The listing builds one solid part. Answer for the finished solid, in the listing's coordinates (mm). Coordinates: 2 decimals unless noted, no trailing zeros. Write each loop counter-clockwise with the first axis right and the second up, starting at its lowest first coordinate (ties: lowest second). Pieces come first, ordered by that corner, then holes. Notation, with made-up numbers: M 8,-17 L 53,-17 A23 ccw 53,-2 Z; hole C 59.25,84 d6. An arc over 180 degrees is marked long. Put each result on its own line as item: value. Start each with the question number.
```python
from build123d import *

# Parameters (mm, degrees)
SKETCH_1_W             = 25
SKETCH_1_H             = 25
SKETCH_1_W_2           = 19
SKETCH_1_H_2           = 19
EXTRUDE_1_DEPTH        = 1285.5
SKETCH_6_R             = 6
CUT_EXTRUDE_1_DEPTH    = 3
PATTERN_LINEAR_1_COUNT = 2
PATTERN_LINEAR_1_PITCH = 1242.5


with BuildPart() as part:
    # 草图1 → 拉伸1 (new body)
    with BuildSketch(Plane.XY):
        with Locations((12.5, -12.5)):
            Rectangle(SKETCH_1_W, SKETCH_1_H)
        with Locations((12.5, -12.5)):
            Rectangle(SKETCH_1_W_2, SKETCH_1_H_2, mode=Mode.SUBTRACT)
    extrude(amount=EXTRUDE_1_DEPTH)

    # 草图4 → Ø6.0 (6) 直径孔1 (revolve, cut)
    with BuildSketch(Plane(origin=(0, -12.5, 1264), x_dir=(0, 0, 1), z_dir=(0, 1, 0))):
        Polygon((0, 0), (0, 31.802581857), (3, 30), (3, 0), align=None)
    hole_wizard_6_0_6_1 = revolve(axis=Axis((-6.35, -12.5, 1264), (1, 0, 0)), mode=Mode.SUBTRACT)

    # 草图6 → 切除-拉伸1 (cut)
    with BuildSketch(Plane.ZY.offset(-25)):
        with Locations(Location((1264, -12.5, 0), (0, 0, 270))):
            Circle(SKETCH_6_R)
    cut_extrude_1 = extrude(amount=CUT_EXTRUDE_1_DEPTH, mode=Mode.SUBTRACT)

    # 阵列(线性)1: Ø6.0 (6) 直径孔1, 切除-拉伸1 ×2
    with Locations(*[(0, 0, -i * PATTERN_LINEAR_1_PITCH) for i in range(1, PATTERN_LINEAR_1_COUNT)]):
        add(hole_wizard_6_0_6_1, mode=Mode.SUBTRACT)
        add(cut_extrude_1, mode=Mode.SUBTRACT)


solid = part.part
```
1) A cutting plane is placed at B-B on z = 116. Write down the section's boundary in (x, y), then the cut area to 3 significant figures.
2) A cutting plane is placed at A-A on x = 15.5. Write down the section's boundary in (y, z).
3) Straight lines are drawn through the part: probe 1 along X at (y, z) = (-8, 510); probe 2 along Y at (x, z) = (21.5, 449); probe 3 along Z at (x, y) = (23.15, -12.5). For each, find the intervals that lie inside material, in ascending order.
4) Given pin 1 Ø15 at (y, z) = (-13, 704.5) entering from -X; pin 2 Ø9.5 at (y, z) = (-12.5, 21.5) entering from +X, each flat-ended and moving along its own axis, determine where each tip first touches the part or whether it passes through.
Answers follow:
1. outline: M 0,-25 L 25,-25 L 25,0 L 0,0 Z; hole M 3,-22 L 22,-22 L 22,-3 L 3,-3 Z
1. area: 264 mm²
2. outline: M -25,0 L -22,0 L -22,1285.5 L -25,1285.5 Z; M -3,0 L 0,0 L 0,1285.5 L -3,1285.5 Z
3. probe 1: x = 0 to 3, 22 to 25
3. probe 2: y = -25 to -22, -3 to 0
3. probe 3: z = 0 to 15.5, 27.5 to 1258, 1270 to 1285.5
4. pin 1: stops at x = 0
4. pin 2: stops at x = 3
